from build123d import *

# Parameters (mm, degrees)
F0_W     = 127
F0_H     = 127
F1_DEPTH = 6.35
F2_R     = 6.35
F3_DEPTH = 27.94


with BuildPart() as f1:
    # F0 (on Front) → F1 (new body, symmetric)
    with BuildSketch(Plane.XZ):
        Rectangle(F0_W, F0_H)
    extrude(amount=F1_DEPTH, both=True)

    # F2 (on Right) → F3 (join, symmetric)
    with BuildSketch(Plane.YZ):
        with Locations((0, 63.5)):
            Circle(F2_R)
    extrude(amount=F3_DEPTH, both=True)


solid = f1.part
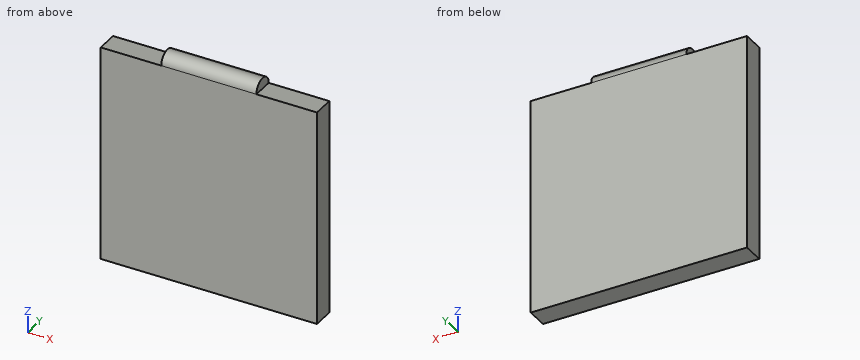
Verification items for the finished model (mm, model axes). Coordinates: 2 decimals unless noted, no trailing zeros. Order: outer loops, then holes, each group sorted by start corner. A loop starts at its lowest first (then second) coordinate and runs counter-clockwise, first axis right, second up.
Item 1: Section check A-A, the plane y = 0. Enter the section's corners in (x, z).
Filled in:
outline: (-63.5, -63.5) - (63.5, -63.5) - (63.5, 63.5) - (27.94, 63.5) - (27.94, 69.85) - (-27.94, 69.85) - (-27.94, 63.5) - (-63.5, 63.5) - close
Item 2: Material ranges on L1, parallel to Z at x = 38, y = 1; L2, parallel to Z at x = -15.5, y = -0.5, recorded low to high.
Filled in:
L1: z = -63.5 to 63.5
L2: z = -63.5 to 69.83
Item 3: Section check B-B, the plane x = -34.5. Enter the section's corners in (y, z), then the cut area to 3 significant figures.
Filled in:
outline: (-6.35, -63.5) - (6.35, -63.5) - (6.35, 63.5) - (-6.35, 63.5) - close
area: 1,610 mm2
Item 4: Depth check by flat-ended pin: pin 1 (4 mm diameter, centred on x = 47, y = 0.5, fed in from +Z); pin 2 (3 mm diameter, centred on y = 0, z = 68, fed in from -X); pin 3 (2 mm diameter, centred on x = -17.5, y = 4, fed in from +Z). Enter the tip coordinate at first touch or a pass-through.
Filled in:
pin 1: stops at z = 63.5
pin 2: stops at x = -27.94
pin 3: stops at z = 69.1
